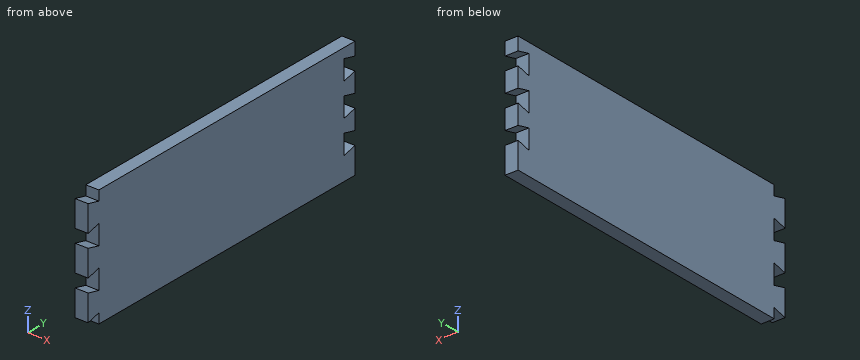
from build123d import *

# Parameters (mm, degrees)
F0_W     = 314.325
F0_H     = 114.3
F1_DEPTH = 12.7
F3_DEPTH = 12.701


with BuildPart() as f1:
    # F0 (on Right) → F1 (new body)
    with BuildSketch(Plane.YZ):
        with Locations((157.1625, 57.15)):
            Rectangle(F0_W, F0_H)
    extrude(amount=F1_DEPTH)

    # F2 (on face) → F3 (cut, through all)
    with BuildSketch(Plane.YZ.offset(12.7)):
        Polygon((12.7, 9.525), (0, 6.358534), (0, 0), (12.7, 0), align=None)
        Polygon((12.7, 47.625), (0, 44.458534), (0, 31.741466), (12.7, 28.575), align=None)
        Polygon((12.7, 85.725), (0, 82.558534), (0, 69.841466), (12.7, 66.675), align=None)
        Polygon((12.7, 104.775), (12.7, 114.3), (0, 114.3), (0, 107.941466), align=None)
        Polygon((314.325, 88.9), (314.325, 101.6), (301.625, 104.766466), (301.625, 85.733534), align=None)
        Polygon((314.325, 57.15), (314.325, 69.85), (301.625, 73.016466), (301.625, 53.983534), align=None)
        Polygon((314.325, 25.4), (314.325, 38.1), (301.625, 41.266466), (301.625, 22.233534), align=None)
    extrude(amount=-F3_DEPTH, mode=Mode.SUBTRACT)


solid = f1.part
Verification items for the finished model (mm, model axes). Round coordinates to 2 decimals unless told otherwise and drop trailing zeros. Loops run counter-clockwise (first coordinate to the right, second up) from the corner with the lowest first, then second, coordinate; pieces in that order, holes last. Notation, with made-up numbers: (30, -0.5) - (38, -0.5) arc R33 ccw to (38, 29.5) - close; hole circle Ø11 at (-24, 41). An arc over 180 degrees is marked (long way). Use one line per item in the form item = value.
1. Gauge pin test, flat end, axial feed: pin 1 Ø4 at (x, z) = (4.5, 75.5) entering from -Y. Record the tip position at first contact, or that the pin passes through.
A:
pin_1 = 12.7
2. Scan lines: probe 1 along Y at (x, z) = (12, 35) (3 decimals); probe 2 along Y at (x, z) = (12, 43) (3 decimals). Record each from-to range of solid material in increasing order.
A:
probe_1 = 12.7 to 301.625
probe_2 = 12.7 to 314.325
3. Section check A-A on x = 6. Record the cut outline in (y, z) (3 decimals), and give its area (3 significant figures).
A:
outline = (0, 6.359) - (12.7, 9.525) - (12.7, 0) - (314.325, 0) - (314.325, 25.4) - (301.625, 22.234) - (301.625, 41.266) - (314.325, 38.1) - (314.325, 57.15) - (301.625, 53.984) - (301.625, 73.016) - (314.325, 69.85) - (314.325, 88.9) - (301.625, 85.734) - (301.625, 104.766) - (314.325, 101.6) - (314.325, 114.3) - (12.7, 114.3) - (12.7, 104.775) - (0, 107.941) - (0, 82.559) - (12.7, 85.725) - (12.7, 66.675) - (0, 69.841) - (0, 44.459) - (12.7, 47.625) - (12.7, 28.575) - (0, 31.741) - close
area = 34,700 mm²
4. Section check B-B on z = 98.5. Record the cut outline in (x, y) (3 decimals), and give its area (3 significant figures).
A:
outline = (0, 0) - (12.7, 0) - (12.7, 301.625) - (0, 301.625) - close
area = 3,830 mm²
